Build history of the part. All positions in model axes, mm. A direction names the side the tool comes from. Round coordinates to 2 decimals unless told otherwise and drop trailing zeros. Write each loop counter-clockwise with the first axis right and the second up, starting at its lowest first coordinate (ties: lowest second). Pieces come first, ordered by that corner, then holes. Notation, with made-up numbers: M 0.25,10 L 4.25,10 A15 ccw 4.25,26 Z; hole C -7,83.5 d4. An arc over 180 degrees is marked long. Write item = value, one per line. Start each with the question number.
Q1. Band-saw the part on C-C on x = -21. Write the cut outline in (y, z), plus the area to 3 significant figures.
Q2. Probe L1, parallel to X at y = -7, z = 100; L2, parallel to Z at x = -18, y = -8.75; L3, parallel to Z at x = -22.5, y = -7.5. List the from-to ranges inside material, lowest first.
Q3. Drop flat-ended pins along their axis: P1, Ø6, axis at x = -13.5, y = -2.5, coming from the +Z side; P2, Ø2, axis at x = 5, z = 102, coming from the +Y side; P3, Ø1, axis at x = -5, y = -3.5, coming from the -Z side; P4, Ø6, axis at x = 10, z = 71, coming from the +Y side. Give the stop position or say it passes through.
Q4. Tool access for faces 1 (the flat face through (31.75, -6, 11)), 2 (the flat face through (4.437, -9, 81)), 3 (the flat face through (-4.432, -10, 81)): list every direction of +Z, -Z, +X, -X, +Y, -Y with a clear straight run to the whole face (end or side of a thin tool).
Q5. Band-saw the part on A-A on x = 0. Write the cut outline in (y, z).
Q6. Band-saw the part on B-B on z = 110. Write the cut outline in (x, y), plus the area to 3 significant figures.
```python
from build123d import *

# Parameters (mm, degrees)
F1_DEPTH = 12.7
F3_DEPTH = 88.9


with BuildPart() as f1:
    # F0 (on Front) → F1 (new body)
    with BuildSketch(Plane.XZ):
        with BuildLine():
            Line((31.75, 37.1686270936), (-31.75, 37.1686270936))
            Line((-31.75, 37.1686270936), (-31.75, -14.7149503491))
            ThreePointArc((-31.75, -14.7149503491), (-31.316464033, -17.0210191569), (-30.0750540643, -19.0122017377))
            Line((-30.0750540643, -19.0122017377), (-4.6750540643, -46.6453007808))
            ThreePointArc((-4.6750540643, -46.6453007808), (0, -48.6980493923), (4.6750540643, -46.6453007808))
            Line((4.6750540643, -46.6453007808), (30.0750540643, -19.0122017377))
            ThreePointArc((30.0750540643, -19.0122017377), (31.316464033, -17.0210191569), (31.75, -14.7149503491))
            Line((31.75, -14.7149503491), (31.75, 37.1686270936))
        make_face()
    extrude(amount=F1_DEPTH)

    # F2 (on face) → F3 (join)
    with BuildSketch(Plane.XY.offset(37.1686270936)):
        with BuildLine():
            Line((-4.4317082143, -6.6040777501), (-4.4317082143, -12.7))
            Line((-4.4317082143, -12.7), (4.4366029292, -12.7))
            Line((4.4366029292, -12.7), (4.4366029292, -6.4954223107))
            ThreePointArc((4.4366029292, -6.4954223107), (0.0543828161, -10.7886524654), (-4.4317082143, -6.6040777501))
        make_face()
        with BuildLine():
            ThreePointArc((4.4366029292, -6.2045776893), (-0.1997650225, -1.9155116264), (-4.4317082143, -6.6040777501))
            ThreePointArc((-4.4317082143, -6.6040777501), (0.0543828161, -10.7886524654), (4.4366029292, -6.4954223107))
            Line((4.4366029292, -6.4954223107), (4.4366029292, -6.2045776893))
        make_face()
    extrude(amount=F3_DEPTH)


solid = f1.part
```
Conclusion:
q1.outline = M -12.7,-28.89 L 0,-28.89 L 0,37.17 L -12.7,37.17 Z
q1.area = 839 mm^2
q2.L1 = -4.43 to 4.44
q2.L2 = -32.15 to 37.17
q2.L3 = -27.25 to 37.17
q3.P1 = 37.17
q3.P2 = -4.43
q3.P3 = -46.83
q3.P4 = through
q4.face_1 = +Z, -Z, +X, +Y, -Y
q4.face_2 = +Z, +X, +Y, -Y
q4.face_3 = +Z, -X, +Y, -Y
q5.outline = M -12.7,-48.7 L 0,-48.7 L 0,37.17 L -1.91,37.17 L -1.91,126.07 L -12.7,126.07 Z
q6.outline = M -4.43,-12.7 L 4.44,-12.7 L 4.44,-6.2 A4.44 ccw long -4.43,-6.6 Z
q6.area = 87.3 mm^2
